from build123d import *

# Parameters (mm, degrees)
SKETCH1_W           = 3
SKETCH1_H           = 1.5
BOSS_EXTRUDE1_DEPTH = 0.75
BOSS_EXTRUDE2_DEPTH = 0.75
SKETCH4_R           = 1.5
SKETCH4_R_2         = 0.7
CUT_EXTRUDE1_DEPTH  = 27.634094691
CUT_EXTRUDE2_DEPTH  = 0.8
FILLET1_R           = 0.5
SKETCH7_R           = 0.6
CUT_EXTRUDE4_DEPTH  = 4


with BuildPart() as part:
    # Sketch1 → Boss-Extrude1 (new, symmetric)
    with BuildSketch(Plane(origin=(0, 0, 0), x_dir=(1, 0, 0), z_dir=(0, 1, 0))):
        Rectangle(SKETCH1_W, SKETCH1_H)
    extrude(amount=BOSS_EXTRUDE1_DEPTH, both=True)

    # Sketch2 → Boss-Extrude2 (add, symmetric)
    with BuildSketch(Plane.XY):
        with BuildLine():
            Line((1.5, 0), (1.5, 18.02350657))
            ThreePointArc((1.5, 18.02350657), (0, 26.25), (-1.5, 18.02350657))
            Line((-1.5, 18.02350657), (-1.5, 0))
            Line((-1.5, 0), (1.5, 0))
        make_face()
    extrude(amount=BOSS_EXTRUDE2_DEPTH, both=True)

    # Sketch4 → Cut-Extrude1 (cut, through all)
    with BuildSketch(Plane.XY.offset(0.75)):
        with Locations((0, 22)):
            Circle(SKETCH4_R)
        with Locations((0, 25.3)):
            Circle(SKETCH4_R_2)
        with Locations((2.857883832, 20.35)):
            Circle(SKETCH4_R_2)
        with Locations((-2.857883832, 20.35)):
            Circle(SKETCH4_R_2)
    extrude(amount=-CUT_EXTRUDE1_DEPTH, mode=Mode.SUBTRACT)

    # Sketch5 → Cut-Extrude2 (cut)
    with BuildSketch(Plane.XY.offset(0.75)):
        with BuildLine():
            Line((0.6, 17.061134616), (0.6, 2.061134616))
            ThreePointArc((0.6, 2.061134616), (0, 1.461134616), (-0.6, 2.061134616))
            Line((-0.6, 2.061134616), (-0.6, 17.061134616))
            ThreePointArc((-0.6, 17.061134616), (0, 17.661134616), (0.6, 17.061134616))
        make_face()
    extrude(amount=-CUT_EXTRUDE2_DEPTH, mode=Mode.SUBTRACT)

    # Fillet1
    fillet1_edges = [part.edges().sort_by_distance(p)[0] for p in [
        (-1.5, -0.75, 0),
        (1.5, -0.75, 0),
    ]]
    fillet(fillet1_edges, radius=FILLET1_R)

    # Sketch7 → Cut-Extrude4 (cut, symmetric)
    with BuildSketch(Plane.XY):
        with Locations((0, 0.227167564)):
            Circle(SKETCH7_R)
    extrude(amount=CUT_EXTRUDE4_DEPTH, both=True, mode=Mode.SUBTRACT)


solid = part.part
Model file for the job. Use its own axes, mm. A direction names the side the tool comes from. Give positions to 0.01 mm unless a question says otherwise; leave off trailing zeros. Loops run counter-clockwise (first coordinate to the right, second up) from the corner with the lowest first, then second, coordinate; pieces in that order, holes last. Notation, with made-up numbers: (66, 88.25) -> (92, 88.25) arc R16 cw to (92, 113.25) -> close; hole circle Ø10 at (63, 23.5). An arc over 180 degrees is marked (long way). Use a Markdown table: item, result. Add a question column.
(1) Wall check: line 1 along Y through (x, z) = (0, -0.35); line 2 along X through (y, z) = (15, 0.4); line 3 along Y through (x, z) = (-0.25, 0.35). Give the ranges that are in metal, low to high.
(2) Tool access for faces 1 (the flat face through (1.5, 9, 0)), 2 (the flat face through (1, 16, 0.75)), 3 (the flat face through (0, 10, -0.05)): list every direction of +Z, -Z, +X, -X, +Y, -Y with a clear straight run to the whole face (end or side of a thin tool).
(3) Slice it at C-C on x = 0. List the corners of the cut face in (y, z), and give its area (3 significant figures).
(4) Mould opens along Y. For faces 4 (the cylindrical face through (0.165, 26.247, 0.01)), 5 (the cylindrical face through (-0.6, 0.25, 0.01)), 6 (the flat face through (-1.5, 9, 0)) say: +Y half, -Y half, draft (parallel to the pull), parting line (faces both ways), or undercut.
(5) Slice it at D-D on z = 0.25. List the corners of the cut face in (x, y).
(6) Slice it at A-A on y = 22. List the corners of the cut face in (x, z), and give its area (3 significant figures).
(7) Drop flat-ended pins along their axis: pin 1 Ø0.6 at (y, z) = (8, 0.5) entering from +X; pin 2 Ø1 at (x, y) = (0, 13.5) entering from +Z. Give the stop position or say it passes through.
(8) Slice it at B-B on x = -2.5. List the corners of the cut face in (y, z), and give its area (3 significant figures).
Filled sheet:
| question | item | result |
|---|---|---|
| 1 | line 1 | -0.75 to -0.37, 0.83 to 20.5, 23.5 to 24.6, 26 to 26.25 |
| 1 | line 2 | -1.5 to -0.6, 0.6 to 1.5 |
| 1 | line 3 | -0.75 to -0.32, 0.77 to 1.52, 17.61 to 20.52, 23.48 to 24.65, 25.95 to 26.24 |
| 2 | face 1 | +Z, -Z, +X, -Y |
| 2 | face 2 | +Z, +X, -X, +Y, -Y |
| 2 | face 3 | +Z |
| 3 | outline | (-0.75, -0.75) -> (-0.37, -0.75) -> (-0.37, 0.75) -> (-0.75, 0.75) -> close; (0.83, -0.75) -> (20.5, -0.75) -> (20.5, 0.75) -> (17.66, 0.75) -> (17.66, -0.05) -> (1.46, -0.05) -> (1.46, 0.75) -> (0.83, 0.75) -> close; (23.5, -0.75) -> (24.6, -0.75) -> (24.6, 0.75) -> (23.5, 0.75) -> close; (26, -0.75) -> (26.25, -0.75) -> (26.25, 0.75) -> (26, 0.75) -> close |
| 3 | area | 19.1 mm2 |
| 4 | face 4 | parting line |
| 4 | face 5 | undercut |
| 4 | face 6 | draft |
| 5 | outline | (-1.5, -0.25) arc R0.5 ccw to (-1, -0.75) -> (1, -0.75) arc R0.5 ccw to (1.5, -0.25) -> (1.5, 18.02) arc R4.25 ccw (long way) to (-1.5, 18.02) -> close; hole circle Ø1.4 at (-2.86, 20.35); hole circle Ø3 at (0, 22); hole circle Ø1.4 at (0, 25.3); hole circle Ø1.2 at (0, 0.23); hole (-0.6, 2.06) arc R0.6 ccw to (0.6, 2.06) -> (0.6, 17.06) arc R0.6 ccw to (-0.6, 17.06) -> close; hole circle Ø1.4 at (2.86, 20.35) |
| 6 | outline | (-4.25, -0.75) -> (-1.5, -0.75) -> (-1.5, 0.75) -> (-4.25, 0.75) -> close; (1.5, -0.75) -> (4.25, -0.75) -> (4.25, 0.75) -> (1.5, 0.75) -> close |
| 6 | area | 8.25 mm2 |
| 7 | pin 1 | x = 1.5 |
| 7 | pin 2 | z = -0.05 |
| 8 | outline | (18.56, -0.75) -> (19.75, -0.75) -> (19.75, 0.75) -> (18.56, 0.75) -> close; (20.95, -0.75) -> (25.44, -0.75) -> (25.44, 0.75) -> (20.95, 0.75) -> close |
| 8 | area | 8.51 mm2 |
